Can you work these out from the model? Positions are in its coordinate system, mm. Give positions to 0.01 mm unless a question says otherwise; leave off trailing zeros. Write each loop counter-clockwise with the first axis right and the second up, starting at its lowest first coordinate (ties: lowest second). Pieces come first, ordered by that corner, then holes. Notation, with made-up numbers: (53, 77) - (78, 77) arc R16 cw to (78, 107) - close; hole circle Ø8 at (77.5, 83). An arc over 180 degrees is marked (long way). Return JSON: item names as keys, results as strings. Group by question number.
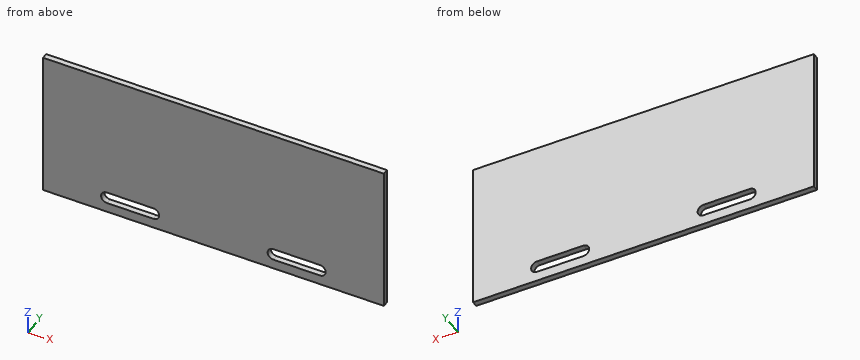
from build123d import *

# Parameters (mm, degrees)
SKETCH1_W               = 1117.6
SKETCH1_H               = 482.6
BOSS_EXTRUDE1_DEPTH     = 9.525
CUT_EXTRUDE1_DEPTH      = 609.971290374
CUT_EXTRUDE1_DEPTH_BACK = 609.971290374


with BuildPart() as part:
    # Sketch1 → Boss-Extrude1 (new, symmetric)
    with BuildSketch(Plane(origin=(0, 0, 0), x_dir=(1, 0, 0), z_dir=(0, 1, 0))):
        Rectangle(SKETCH1_W, SKETCH1_H)
    extrude(amount=BOSS_EXTRUDE1_DEPTH, both=True)

    # Sketch2 → Cut-Extrude1 (cut, two sides: drawn at the far end of the back side and taken through both)
    with BuildSketch(Plane.XZ.offset(9.525).offset(-CUT_EXTRUDE1_DEPTH_BACK)):
        with BuildLine():
            Line((-349.25, -171.45), (-196.85, -171.45))
            ThreePointArc((-196.85, -171.45), (-177.8, -190.5), (-196.85, -209.55))
            Line((-196.85, -209.55), (-349.25, -209.55))
            ThreePointArc((-349.25, -209.55), (-368.3, -190.5), (-349.25, -171.45))
        make_face()
        with BuildLine():
            Line((196.85, -171.45), (349.25, -171.45))
            ThreePointArc((349.25, -171.45), (368.3, -190.5), (349.25, -209.55))
            Line((349.25, -209.55), (196.85, -209.55))
            ThreePointArc((196.85, -209.55), (177.8, -190.5), (196.85, -171.45))
        make_face()
    extrude(amount=CUT_EXTRUDE1_DEPTH + CUT_EXTRUDE1_DEPTH_BACK, mode=Mode.SUBTRACT)


solid = part.part
1) Imagine slicing it at A-A, the plane z = -190.5. Write out the boundary of the cut face in (x, y) (3 decimals).
2) I need wall thicknesses on line 1 along X through (y, z) = (-8, -193); line 2 along X through (y, z) = (0, -200); line 3 along Z through (x, y) = (-257.5, 6.75). Which ranges of each line are inside material? Lowest first, please.
3) Imagine slicing it at B-B, the plane y = -2.75. Write out the boundary of the cut face in (x, z), and give its area (3 significant figures).
Resolved:
{
 "1": {"outline": "(-558.8, -9.525) - (-368.3, -9.525) - (-368.3, 9.525) - (-558.8, 9.525) - close; (-177.8, -9.525) - (177.8, -9.525) - (177.8, 9.525) - (-177.8, 9.525) - close; (368.3, -9.525) - (558.8, -9.525) - (558.8, 9.525) - (368.3, 9.525) - close"},
 "2": {"line 1": "-558.8 to -368.14, -177.96 to 177.96, 368.14 to 558.8", "line 2": "-558.8 to -365.76, -180.34 to 180.34, 365.76 to 558.8", "line 3": "-241.3 to -209.55, -171.45 to 241.3"},
 "3": {"outline": "(-558.8, -241.3) - (558.8, -241.3) - (558.8, 241.3) - (-558.8, 241.3) - close; hole (-349.25, -209.55) - (-196.85, -209.55) arc R19.05 ccw to (-196.85, -171.45) - (-349.25, -171.45) arc R19.05 ccw to start; hole (196.85, -209.55) - (349.25, -209.55) arc R19.05 ccw to (349.25, -171.45) - (196.85, -171.45) arc R19.05 ccw to start", "area": "525,000 mm^2"}
}
